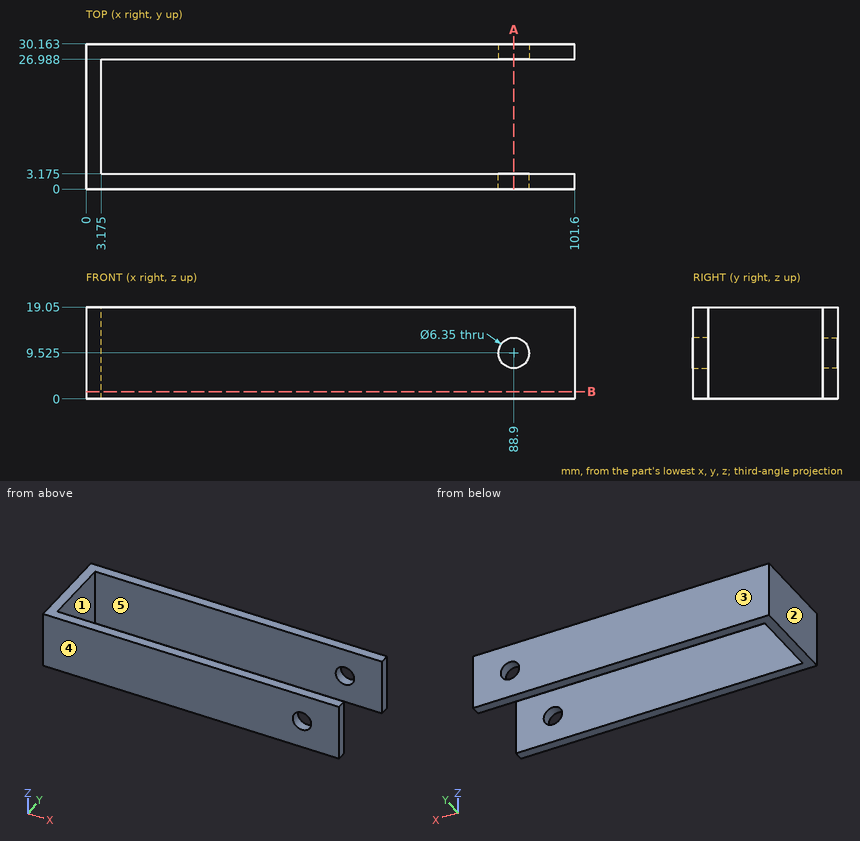
Study the drawing (mm; zero at the part's minimum x, y, z) and answer. A direction names the side the tool comes from. Give positions to 0.01 mm unless a question says otherwise; leave off trailing zeros. Loops run counter-clockwise (first coordinate to the right, second up) from the corner with the lowest first, then second, coordinate; pieces in that order, holes last. Notation, with made-up numbers: M 18.5,-28 L 26.5,-28 A5 ccw 26.5,-22 Z; hole C 80.5,49.5 d10. An arc over 180 degrees is marked long. Use CSV: the item, a comma, the result in double quotes.
1) Find section B-B on z = 1.5. Write down the section's boundary in (x, y) (1 decimal).
Answer:
outline,"M 0,0 L 101.6,0 L 101.6,3.2 L 3.2,3.2 L 3.2,27 L 101.6,27 L 101.6,30.2 L 0,30.2 Z"
2) Determine the mould class of the marked faces 1, 2 and 3 for opening direction Y: released by +Y, released by -Y, zero draft, split by the parting line, or undercut.
Answer:
face 1,"undercut"
face 2,"zero draft"
face 3,"released by +Y"
3) Which of the six approach directions +Z, -Z, +X, -X, +Y, -Y give full straight-line access (tool end or side, diameter ignored) to the marked faces 4 and 5?
Answer:
face 4,"+Z, -Z, +X, -X, -Y"
face 5,"+Z, -Z, +X"
4) Find section A-A on x = 88.9. Give the number of separate pieces and of enclosed holes in the cut face.
Answer:
separate pieces,"4"
enclosed holes,"0"
5) Consider L1, parallel to Z at x = 88.9, y = 28.5; L2, parallel to Y at x = 65.5, z = 14.5 (1 decimal); L3, parallel to X at y = 24.5, z = 17.75 (1 decimal). Determine where each line is inside the solid, lowest interval first.
Answer:
L1,"0 to 6.35, 12.7 to 19.05"
L2,"0 to 3.2, 27 to 30.2"
L3,"0 to 3.2"
6) Given P1, Ø12, axis at x = 64, y = 17, coming from the +Z side; P2, Ø4, axis at y = 14.5, z = 9, coming from the +X side (1 decimal), each flat-ended and moving along its own axis, determine where each tip first touches the part or whether it passes through.
Answer:
P1,"through"
P2,"x = 3.2"
